Check sheet for the modelled part. Datum: model origin and axes. Units: mm. A direction names the side the tool comes from. Give positions to 0.01 mm unless a question says otherwise; leave off trailing zeros. Order: outer loops, then holes, each group sorted by start corner. A loop starts at its lowest first (then second) coordinate and runs counter-clockwise, first axis right, second up.
Item 1: Material ranges on line 1 along X through (y, z) = (0, 14.5); line 2 along X through (y, z) = (-17, 12); line 3 along Y through (x, z) = (10.5, 22.5), recorded low to high.
Item 2: Access from +Z, -Z, +X, -X, +Y, -Y to the whole of each face (thin tool, end or side, straight path). Record for faces 1 (the flat face through (23, 16.801, 17)), 2 (the flat face through (5, -17.9, 11)), 3 (the flat face through (11.5, 0.5, 17)), 4 (the flat face through (-23, -16.801, 17)), 5 (the cylindrical face through (2.764, -12.447, 3.451)).
Item 3: Sectioned sample at B-B on z = 12. Count the separate pieces of the cut face and the enclosed holes in it, and give its area (3 significant figures).
Item 4: Gauge pin test, flat ends, axial feed: P1, Ø17, axis at x = 0, y = 0, coming from the -Z side; P2, Ø1, axis at x = -8, z = 8, coming from the -Y side; P3, Ø4, axis at y = 23.5, z = 23.5, coming from the -X side. Record the tip position at first contact, or that the pin passes through.
Item 5: Sectioned sample at A-A on z = 30.5. Record the boundary of the cut face in (x, y).
Item 6: Release check for a two-part mould opening along X. For faces 6 (the flat face through (-23, 16.801, 17)), 7 (the flat face through (-16.801, 23, 17)), 8 (the cylindrical face through (-1.63, 15.76, 24.22)) record: released by +X, released by -X, zero draft, split by the parting line, or undercut.
Autodesk Inventor part; units mm, degrees
ref_plane "Work Plane2" through (-27.39, -0.0644, 16.8356) normal (0, -0.7071, -0.7071) x (0, 0.7071, -0.7071)
ref_plane "Work Plane3" through (-16.9, 21.1423, 33.8) normal (0, 0, -1) x (0, 1, 0)
ref_plane "YZ Plane" through (0, 0, 0) normal (1, 0, 0) x (0, 1, 0)
sketch "Sketch1" plane through (0, 0, 0) normal (0, 0, 1) x (1, 0, 0)
  line L0 (-34.86, 0) -> (34.86, 0) construction
  line L1 (0, -34.86) -> (0, 34.86) construction
  line L2 (0, 0) -> (16.9726, 16.9726) construction
  line L3 (0, 0) -> (24.0028, 0) construction
  line L4 (0, 24.9) -> (16.8009, 24.9)
  line L5 (16.8009, 24.9) -> (16.8009, 21.2415)
  line L6 (16.8009, 21.2415) -> (19.0212, 19.0212)
  line L7 (24.9, 0) -> (24.9, 16.8009)
  line L8 (24.9, 16.8009) -> (21.2415, 16.8009)
  line L9 (21.2415, 16.8009) -> (19.0212, 19.0212)
  line L10 (0, -24.9) -> (16.8009, -24.9)
  line L11 (16.8009, -24.9) -> (16.8009, -21.2415)
  line L12 (16.8009, -21.2415) -> (19.0212, -19.0212)
  line L13 (24.9, 0) -> (24.9, -16.8009)
  line L14 (24.9, -16.8009) -> (21.2415, -16.8009)
  line L15 (21.2415, -16.8009) -> (19.0212, -19.0212)
  line L16 (0, 0) -> (-16.9726, 16.9726) construction
  line L17 (0, 0) -> (-24.0028, 0) construction
  line L18 (0, 24.9) -> (-16.8009, 24.9)
  line L19 (-16.8009, 24.9) -> (-16.8009, 21.2415)
  line L20 (-16.8009, 21.2415) -> (-19.0212, 19.0212)
  line L21 (-24.9, 0) -> (-24.9, 16.8009)
  line L22 (-24.9, 16.8009) -> (-21.2415, 16.8009)
  line L23 (-21.2415, 16.8009) -> (-19.0212, 19.0212)
  line L24 (0, -24.9) -> (-16.8009, -24.9)
  line L25 (-16.8009, -24.9) -> (-16.8009, -21.2415)
  line L26 (-16.8009, -21.2415) -> (-19.0212, -19.0212)
  line L27 (-21.2415, -16.8009) -> (-19.0212, -19.0212)
  line L28 (-24.9, -16.8009) -> (-21.2415, -16.8009)
  line L29 (-24.9, 0) -> (-24.9, -16.8009)
  circle A0 centre (0, 0) radius 7.5
  dimension "d17" = 45
  dimension "d18" = 24.9
  dimension "d20" = 3.14
  dimension "d21" = 26.9
  dimension "d22" = 15
extrude "Extrusion1" add sketch "Sketch1" along normal blind 3
sketch "Sketch6" plane through (0, 0, 3) normal (0, 0, 1) x (1, 0, 0)
  circle A0 centre (0, 0) radius 7.5
  line L0 (16.8009, 24.9) -> (-16.8009, 24.9)
  line L1 (-16.8009, 24.9) -> (-16.8009, 21.2415)
  line L2 (-16.8009, 21.2415) -> (-21.2415, 16.8009)
  line L3 (-21.2415, 16.8009) -> (-24.9, 16.8009)
  line L4 (-24.9, 16.8009) -> (-24.9, -16.8009)
  line L5 (-24.9, -16.8009) -> (-21.2415, -16.8009)
  line L6 (-21.2415, -16.8009) -> (-16.8009, -21.2415)
  line L7 (-16.8009, -21.2415) -> (-16.8009, -24.9)
  line L8 (-16.8009, -24.9) -> (16.8009, -24.9)
  line L9 (16.8009, -24.9) -> (16.8009, -21.2415)
  line L10 (16.8009, -21.2415) -> (21.2415, -16.8009)
  line L11 (21.2415, -16.8009) -> (24.9, -16.8009)
  line L12 (24.9, -16.8009) -> (24.9, 16.8009)
  line L13 (24.9, 16.8009) -> (21.2415, 16.8009)
  line L14 (21.2415, 16.8009) -> (16.8009, 21.2415)
  line L15 (16.8009, 21.2415) -> (16.8009, 24.9)
  line L16 (24.9, -16.8009) -> (24.9, 16.8009)
  line L17 (24.9, 13.5502) -> (-24.9, 13.5502)
  line L18 (-24.9, 16.8009) -> (-24.9, -16.8009)
ref_plane "Work Plane2" through (-27.39, -0.0644, 16.8356) normal (0, -0.7071, -0.7071) x (0, 0.7071, -0.7071)
extrude "Extrusion6" add sketch "Sketch6" along normal up to surface contours L12 L11 L10 L9 L8 L7 L6 L5 L4 L17 surface through (-27.39, -0.0644, 16.8356) normal (0, -0.7071, -0.7071)
sketch "Sketch7" plane through (-16.8009, -24.9, 0) normal (0, -1, 0) x (1, 0, 0)
  line L0 (-0.0991, 33.8) -> (0.8009, 33.8)
  arc A0 (-6.0991, 41.8) -> (-8.0991, 39.8) centre (-6.0991, 39.8) ccw
  arc A1 (41.7009, 39.8) -> (39.7009, 41.8) centre (39.7009, 39.8) ccw
  line L1 (41.9057, 41.8) -> (-10.6447, 41.8)
  line L2 (-10.6447, 41.8) -> (-10.6447, 33.8)
  line L3 (-10.6447, 33.8) -> (41.9057, 33.8)
  line L4 (41.9057, 33.8) -> (41.9057, 41.8)
  point P0 (16.8009, 0)
extrude "Extrusion7" cut sketch "Sketch7" against normal through all
sketch "Sketch8" plane through (21.2415, -16.8009, 0) normal (0, -1, 0) x (1, 0, 0)
  line L0 (-8.7415, 0) -> (-33.7415, 0)
  line L1 (-33.7415, -1) -> (-8.7415, -1)
  line L2 (-46.1415, 33.572) -> (-42.483, 33.572)
  line L3 (3.6585, 33.8) -> (0.0423, 33.8)
  line L4 (0, 33.572) -> (3.6585, 33.572)
  line L5 (-46.1415, 3.2209) -> (-46.1415, 33.572)
  line L6 (3.6585, 33.572) -> (-46.1415, 33.572)
  line L7 (-46.1415, 33.572) -> (-46.1415, 30.572)
  line L8 (-46.1415, 30.572) -> (3.6585, 30.572)
  line L9 (3.6585, 30.572) -> (3.6585, 33.572)
  dimension "d45" = 3
sketch "Sketch9" plane through (-16.8009, -24.9, 0) normal (0, -1, 0) x (1, 0, 0)
  line L0 (33.7009, 0) -> (33.0009, 0) construction
  line L1 (36.0327, -6) -> (22.7009, -6) construction
  circle A0 centre (16.8009, 16.9) radius 16.9 construction
  circle A1 centre (16.8009, 16.9) radius 7.5
  line L2 (39.7009, 8.1978) -> (33.7009, 8.1978)
  line L3 (33.7009, 8.1978) -> (33.7009, 0)
  line L4 (33.0009, 0) -> (33.0009, -3.7)
  line L5 (33.0009, -3.7) -> (22.7009, -3.7)
  line L6 (22.7009, -3.7) -> (22.7009, -6)
  arc A2 (39.7009, -2.3319) -> (36.0327, -6) centre (36.8009, -3.1) ccw
  line L7 (39.7009, 8.1978) -> (39.7009, -2.3319)
  point P0 (16.8009, 0)
  dimension "d46" = 15
extrude "Extrusion8" cut sketch "Sketch9" against normal through all
sketch "Sketch10" plane through (-16.8009, -24.9, 0) normal (0, -1, 0) x (1, 0, 0)
  circle A0 centre (16.8009, 16.9) radius 7.5
  circle A1 centre (16.8009, 16.9) radius 12.75
  point P0 (16.8009, 0)
  dimension "d49" = 25.5
extrude "Extrusion9" cut sketch "Sketch10" against normal blind 7
sketch "Sketch11" plane through (0, 0, 0) normal (0, 0, -1) x (-1, 0, 0)
  circle A0 centre (0, 0) radius 7.5
  circle A1 centre (0, 0) radius 12.75
  dimension "d52" = 25.5
extrude "Extrusion10" cut sketch "Sketch11" against normal blind 7
sketch "Sketch12" plane through (-24.9, 13.5502, 3.2209) normal (0, 0.7071, 0.7071) x (1, 0, 0)
  line L0 (32.9, -31.2053) -> (32.9, -6.2053) construction
  line L1 (32.9, -6.2053) -> (16.9, -6.2053) construction
  line L2 (16.9, -6.2053) -> (16.9, -31.2053) construction
  line L3 (16.9, -31.2053) -> (32.9, -31.2053) construction
  line L4 (32.9, -31.2053) -> (16.9, -31.2053) construction
  line L5 (16.9, -31.2053) -> (16.9, -6.2053) construction
  line L6 (16.9, -6.2053) -> (32.9, -6.2053) construction
  line L7 (32.9, -6.2053) -> (32.9, -31.2053) construction
  line L8 (16.4, -5.7053) -> (33.4, -5.7053)
  line L9 (33.4, -5.7053) -> (33.4, -31.7053)
  line L10 (33.4, -31.7053) -> (16.4, -31.7053)
  line L11 (16.4, -31.7053) -> (16.4, -5.7053)
  line L12 (36.4, -2.7053) -> (13.4, -2.7053)
  line L13 (13.4, -2.7053) -> (13.4, -34.7053)
  line L14 (13.4, -34.7053) -> (36.4, -34.7053)
  line L15 (36.4, -34.7053) -> (36.4, -2.7053)
  point P0 (24.9, -7.3039)
  dimension "d55" = 0.5
  dimension "d56" = 3
extrude "Extrusion11" add sketch "Sketch12" along normal blind 1
sketch "Sketch13" plane through (0, 0, 3) normal (0, 0, 1) x (1, 0, 0)
  line L0 (-24.9, 13.5502) -> (24.9, 13.5502)
  line L1 (24.9, 13.5502) -> (24.9, 16.8009)
  line L2 (24.9, 16.8009) -> (21.2415, 16.8009)
  line L3 (21.2415, 16.8009) -> (16.8009, 21.2415)
  line L4 (16.8009, 21.2415) -> (16.8009, 24.9)
  line L5 (16.8009, 24.9) -> (-16.8009, 24.9)
  line L6 (-16.8009, 24.9) -> (-16.8009, 21.2415)
  line L7 (-16.8009, 21.2415) -> (-21.2415, 16.8009)
  line L8 (-21.2415, 16.8009) -> (-24.9, 16.8009)
  line L9 (-24.9, 16.8009) -> (-24.9, 13.5502)
  point P0 (0, 0)
ref_plane "Work Plane3" through (-16.9, 21.1423, 33.8) normal (0, 0, -1) x (0, 1, 0)
extrude "Extrusion12" add sketch "Sketch13" along normal up to surface (30.8 mm away)
sketch "Sketch14" plane through (-16.8009, 24.9, 0) normal (0, 1, 0) x (1, 0, 0)
  line L0 (-0.0991, -33.8) -> (-0.0991, 0) construction
  line L1 (33.6017, -33.8) -> (0, -33.8)
  line L2 (0, 0) -> (33.6017, 0)
  line L3 (33.6017, 0) -> (33.6017, -33.8)
  arc A0 (9.3011, -16.8356) -> (24.3006, -16.8356) centre (16.8009, -16.9) ccw construction
  circle A1 centre (16.8009, -16.9) radius 12.75
  point P0 (16.8009, 0)
  dimension "d61" = 25.5
extrude "Extrusion13" cut sketch "Sketch14" against normal blind 7
sketch "Sketch15" plane through (0, 17.9, 16.9) normal (0, 1, 0) x (1, 0, 0)
  circle A0 centre (0, 0) radius 7.5
  point P0 (0, 16.9)
extrude "Extrusion14" cut sketch "Sketch15" against normal through all
sketch "Sketch16" plane through (21.2415, -16.8009, 33.572) normal (0, 0.7071, 0.7071) x (1, 0, 0)
  line L0 (-42.255, -0.3224) -> (-0.228, -0.3224)
  line L1 (-0.228, -0.3224) -> (0, 0)
  line L2 (0, 0) -> (3.6585, 0)
  line L3 (3.6585, 0) -> (3.6585, 42.9229)
  line L4 (3.6585, 42.9229) -> (-46.1415, 42.9229)
  line L5 (-46.1415, 42.9229) -> (-46.1415, 0)
  line L6 (-46.1415, 0) -> (-42.483, 0)
  line L7 (-42.483, 0) -> (-42.255, -0.3224)
  ellipse E0 centre (-21.2415, 23.76) end of major axis (-21.2415, 41.7912) minor radius 12.75 (-16.0323, 40.2176) -> (-26.4507, 40.2176) ccw
  line L8 (-9.7415, 40.2176) -> (-9.7415, 8.2176)
  line L9 (-9.7415, 8.2176) -> (-32.7415, 8.2176)
  line L10 (-32.7415, 8.2176) -> (-32.7415, 40.2176)
  line L11 (-16.0323, 40.2176) -> (-9.7415, 40.2176)
  line L12 (-4.4406, 18.0121) -> (-38.0423, 18.0121)
  circle A0 centre (-35.0423, 18.0121) radius 1.4
  circle A1 centre (-7.4406, 18.0121) radius 1.4
  line L13 (-32.7415, 40.2176) -> (-26.4507, 40.2176)
  point P0 (-21.2415, 35.619)
  point P1 (-4.4406, 18.0121)
  dimension "d66" = 3
  dimension "d67" = 3
  dimension "d68" = 2.8
  dimension "d69" = 2.8
extrude "Extrusion15" cut sketch "Sketch16" along normal through all both and the other way through all contours A1 L12 | L12 A1 | A0 L12 | L12 A0
sketch "Sketch17" plane through (-24.9, -16.8009, 0) normal (-1, 0, 0) x (0, 0, 1)
  line L0 (43.2726, 50.002) -> (33.5, 50.002)
  line L1 (33.5, 50.002) -> (33.5, -21.818)
  line L2 (33.5, -21.818) -> (43.2726, -21.818)
  line L3 (43.2726, -21.818) -> (43.2726, 50.002)
  line L4 (0, 0) -> (0, 33.6017)
  point P0 (0, 16.8009)
  dimension "d72" = 33.5
extrude "Extrusion16" cut sketch "Sketch17" against normal through all
sketch "Sketch18" plane through (-24.9, 13.5502, 33.5) normal (0, 0, 1) x (1, 0, 0)
  line L0 (49.8, 0) -> (0, 0)
  line L1 (49.8, 3.2506) -> (49.8, 0)
  line L2 (46.1415, 3.2506) -> (49.8, 3.2506)
  line L3 (41.7009, 7.6912) -> (46.1415, 3.2506)
  line L4 (41.7009, 11.3498) -> (41.7009, 7.6912)
  line L5 (8.0991, 11.3498) -> (41.7009, 11.3498)
  line L6 (8.0991, 7.6912) -> (8.0991, 11.3498)
  line L7 (3.6585, 3.2506) -> (8.0991, 7.6912)
  line L8 (0, 3.2506) -> (3.6585, 3.2506)
  line L9 (0, 0) -> (0, 3.2506)
  line L10 (3.6585, -30.3511) -> (0, -30.3511)
  line L11 (8.0991, -34.7917) -> (3.6585, -30.3511)
  line L12 (8.0991, -38.4502) -> (8.0991, -34.7917)
  line L13 (41.7009, -38.4502) -> (8.0991, -38.4502)
  line L14 (41.7009, -34.7917) -> (41.7009, -38.4502)
  line L15 (46.1415, -30.3511) -> (41.7009, -34.7917)
  line L16 (49.8, -30.3511) -> (46.1415, -30.3511)
  line L17 (49.8, -30.2791) -> (49.8, -30.3511)
  line L18 (0, -30.2791) -> (49.8, -30.2791)
  line L19 (0, -30.3511) -> (0, -30.2791)
  line L20 (41.7009, 7.6912) -> (46.1415, 3.2506) construction
  line L21 (43.9212, 5.4709) -> (5.8788, -32.5714) construction
  line L22 (8.0991, -34.7917) -> (3.6585, -30.3511) construction
  circle A0 centre (43.9212, 5.4709) radius 2.5
  point P0 (24.9, -13.5502)
  dimension "d75" = 5
extrude "Extrusion17" cut sketch "Sketch18" against normal through all contours A0 L3 | L3 A0
mirror "Mirror3" about plane through (0, 0, 0) normal (1, 0, 0) of "Extrusion17"
mirror "Mirror4" about plane through (0, 0, 0) normal (0, 1, 0) of "Extrusion17", "Mirror3"
pattern_circular "Circular Pattern1" count 4 over 360 about axis through (0, -24.9, 16.9) along (0, 1, 0) of "Extrusion17", "Mirror3", "Mirror4"
properties part number "20_Cube_Insert_Beamsplitter"
Report:
1. line 1: x = -24.9 to -7.5, 7.5 to 24.9
1. line 2: x = -21.04 to -20.49, -17.55 to -5.68, 5.68 to 17.55, 20.49 to 21.04
1. line 3: y = -17.9 to -4.31, 13.55 to 17.9
2. face 1: +Z, -Z, +X, +Y
2. face 2: -Y
2. face 3: +Z, +X
2. face 4: +Z, -Z, -X, -Y
2. face 5: -Z
3. separate pieces: 4
3. enclosed holes: 2
3. area: 1,110 mm2
4. P1: stops at z = 7
4. P2: stops at y = -17.9
4. P3: stops at x = -16.8
5. outline: (-24.9, -16.8) - (-21.24, -16.8) - (-20.79, -17.25) arc R2.5 cw to (-17.25, -20.79) - (-16.8, -21.24) - (-16.8, -24.9) - (16.8, -24.9) - (16.8, -21.24) - (17.25, -20.79) arc R2.5 cw to (20.79, -17.25) - (21.24, -16.8) - (24.9, -16.8) - (24.9, -13.73) - (-24.9, -13.73) - close; (-24.9, 13.55) - (24.9, 13.55) - (24.9, 16.8) - (21.24, 16.8) - (20.79, 17.25) arc R2.5 cw to (17.25, 20.79) - (16.8, 21.24) - (16.8, 24.9) - (-16.8, 24.9) - (-16.8, 21.24) - (-17.25, 20.79) arc R2.5 cw to (-20.79, 17.25) - (-21.24, 16.8) - (-24.9, 16.8) - close
6. face 6: zero draft
6. face 7: released by -X
6. face 8: undercut
